Here's the drawing with two shaded views (mm, measured from the low corner). I have some questions. A direction names the side the tool comes from. Coordinates: 2 decimals unless noted, no trailing zeros. Order: outer loops, then holes, each group sorted by start corner. A loop starts at its lowest first (then second) coordinate and runs counter-clockwise, first axis right, second up. Notation, with made-up numbers: (25.5, -1.5) -> (66.5, -1.5) arc R14 cw to (66.5, 13.5) -> close; hole circle Ø2 at (45.5, 80). An arc over 180 degrees is marked (long way). Return JSON: item names as keys, results as strings. Group by question number.
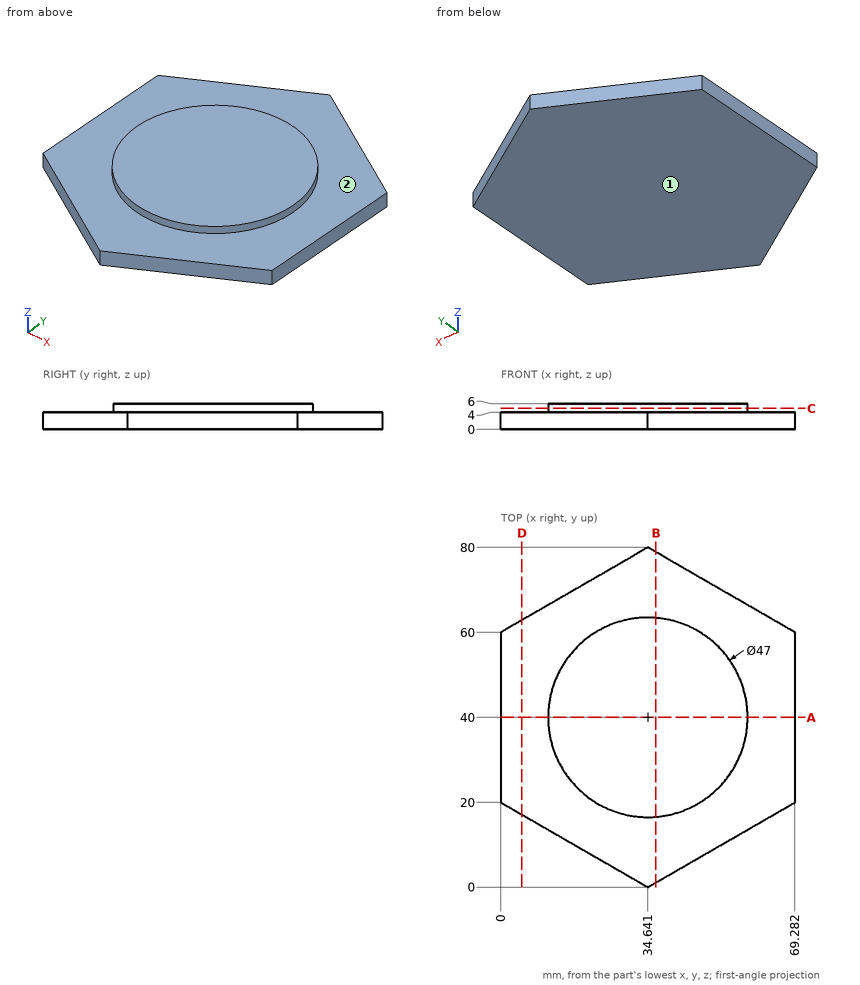
Q1. I want a section at D-D on x = 5. Please give me the cut outline in (y, z).
Q2. On a 3-axis mill with a long thin cutter (end or side, diameter ignored), from which of +Z, -Z, +X, -X, +Y, -Y can I reach the whole of each face in a straight line? I mean the marked faces 1 and 2. Say none if no direction works.
Q3. I want a section at B-B on x = 36.5. Please give me the cut outline in (y, z).
Q4. I want a section at A-A on y = 40. Please give me the cut outline in (x, z), and give its area (3 significant figures).
Q5. I'm going to push flat-ended pins straight in: pin 1 Ø2 at (y, z) = (15.5, 1) entering from +X; pin 2 Ø3 at (x, y) = (25, 38.5) entering from -Z; pin 3 Ø5 at (x, y) = (62, 14) entering from +Z; pin 4 Ø1 at (x, z) = (56.5, 3.5) entering from +Y. Where does each tip first touch, or does it pass through?
Q6. I want a section at C-C on z = 4.95. Please give me the cut outline in (x, y).
Q7. I need wall thicknesses on line 1 along Z through (x, y) = (7.5, 48); line 2 along X through (y, z) = (29.5, 5.5); line 3 along Y through (x, z) = (27, 1.4). Which ranges of each line are inside material? Lowest first, please. Write a range as from..to.
Response values:
{
 "1": {"outline": "(17.11, 0) -> (62.89, 0) -> (62.89, 4) -> (17.11, 4) -> close"},
 "2": {"face 1": "-Z, +X, -X, +Y, -Y", "face 2": "+Z"},
 "3": {"outline": "(1.07, 0) -> (78.93, 0) -> (78.93, 4) -> (63.43, 4) -> (63.43, 6) -> (16.57, 6) -> (16.57, 4) -> (1.07, 4) -> close"},
 "4": {"outline": "(0, 0) -> (69.28, 0) -> (69.28, 4) -> (58.14, 4) -> (58.14, 6) -> (11.14, 6) -> (11.14, 4) -> (0, 4) -> close", "area": "371 mm²"},
 "5": {"pin 1": "stops at x = 63.22", "pin 2": "stops at z = 0", "pin 3": "stops at z = 4", "pin 4": "stops at y = 67.67"},
 "6": {"outline": "circle Ø47 at (34.64, 40)"},
 "7": {"line 1": "z = 0..4", "line 2": "x = 13.62..55.66", "line 3": "y = 4.41..75.59"}
}
